Build history of the part. All positions in model axes, mm. A direction names the side the tool comes from. Give positions to 0.01 mm unless a question says otherwise; leave off trailing zeros. Write each loop counter-clockwise with the first axis right and the second up, starting at its lowest first coordinate (ties: lowest second). Pieces come first, ordered by that corner, then holes. Notation, with made-up numbers: (-12.5, 64) -> (4.5, 64) arc R22 ccw to (4.5, 73) -> close; hole circle Ø1 at (52, -27.5). An arc over 180 degrees is marked (long way). Write item = value, one per line. Start each with the question number.
Q1. Saw through at A-A, the plane y = 2. List the corners of the cut face in (x, z).
Q2. Drop flat-ended pins along their axis: P1, Ø5, axis at y = 3.5, z = -31, coming from the +X side; P2, Ø5, axis at y = 2.5, z = -21.5, coming from the -X side; P3, Ø1.5, axis at x = -8, z = -12.5, coming from the -Y side. Give the stop position or say it passes through.
Q3. Tool access for faces 1 (the face through (-5.26, 11.52, -18.68)), 2 (the face through (-20, 5, -3)), 3 (the face through (-42.05, 4.93, -3.43)), 4 (the face through (-36.238, 1.479, -29.956)), 5 (the face through (-42.07, 4.93, -46.55)): list every direction of +Z, -Z, +X, -X, +Y, -Y with a clear straight run to the whole face (end or side of a thin tool).
Q4. Mould opens along X. For faces 6 (the face through (-29.04, 1.48, -8.59)), 7 (the face through (-43.45, 11.52, -48)), 8 (the face through (-15, 13, -9)) say: pulls with the +X half, pulls with the -X half, needs draft (parallel to the pull), parting line crosses it, or undercut.
Q5. Wall check: line 1 (X direction, y = 3.25, z = -25); line 2 (Z direction, x = -20.5, y = 12.2); line 3 (Z direction, x = -20.5, y = 5.5). Give the ranges that are in metal, low to high.
Q6. Saw through at D-D, the plane y = 7. List the corners of the cut face in (x, z).
Q7. Saw through at B-B, the plane x = -20.5. List the corners of the cut face in (y, z), then the cut area to 3 significant figures.
Q8. Saw through at C-C, the plane z = -25. List the corners of the cut face in (x, y).
Autodesk Inventor part; units mm, degrees
ref_plane "YZ Plane" through (0, 0, 0) normal (1, 0, 0) x (0, 1, 0)
ref_plane "XZ Plane" through (0, 0, 0) normal (0, 1, 0) x (-1, 0, 0)
ref_plane "XY Plane" through (0, 0, 0) normal (0, 0, 1) x (1, 0, 0)
sketch "Эскиз1" plane through (0, 0, 0) normal (0, 1, 0) x (-1, 0, 0)
  arc A0 (41, -50) -> (45.5, -45.5) centre (41, -45.5) ccw
  line L0 (0, -50) -> (41, -50)
  arc A1 (-4.5, -45.5) -> (0, -50) centre (0, -45.5) ccw
  line L1 (-4.5, -4.5) -> (-4.5, -45.5)
  arc A2 (0, 0) -> (-4.5, -4.5) centre (0, -4.5) ccw
  line L2 (-1.5, -45.5) -> (-1.5, -4.5)
  arc A3 (0, -3) -> (-1.5, -4.5) centre (0, -4.5) ccw
  line L3 (0, -3) -> (41, -3)
  line L4 (41, 0) -> (0, 0)
  arc A4 (45.5, -4.5) -> (41, 0) centre (41, -4.5) ccw
  line L5 (45.5, -45.5) -> (45.5, -4.5)
  line L6 (42.5, -4.5) -> (42.5, -45.5)
  arc A5 (42.5, -4.5) -> (41, -3) centre (41, -4.5) ccw
  line L7 (41, -47) -> (0, -47)
  arc A6 (41, -47) -> (42.5, -45.5) centre (41, -45.5) ccw
  arc A7 (-1.5, -45.5) -> (0, -47) centre (0, -45.5) ccw
  circle A8 centre (20.5, -25) radius 18.5
  circle A9 centre (20.5, -25) radius 16.5
  circle A10 centre (20.5, -25) radius 14.5
  circle A11 centre (20.5, -25) radius 13.5
  point P0 (11.5, -30)
extrude "Выдавливание1" add sketch "Эскиз1" along normal blind 10 contours L2 A3 L3 A5 L6 A6 L7 A7 | A8 | A9 | A10 | A11
extrude "Выдавливание2" cut sketch "Эскиз1" along normal blind 3 contours A8 | A10
extrude "Выдавливание3" cut sketch "Эскиз1" along normal blind 14.75 contours A10 | A11
extrude "Выдавливание4" add sketch "Эскиз1" along normal blind 13 contours L0 A1 L1 A2 L4 A4 L5 A0
extrude "Выдавливание5" add sketch "Эскиз1" along normal blind 13 contours L2 A3 L3 A5 L6 A6 L7 A7 | A8 | A9 | A10 | A11
extrude "Выдавливание6" cut sketch "Эскиз1" along normal blind 10 contours L0 A1 L1 A2 L4 A4 L5 A0
extrude "Выдавливание7" cut sketch "Эскиз1" along normal blind 3 contours A8 | A10
extrude "Выдавливание8" cut sketch "Эскиз1" along normal blind 15 contours A10 | A11
sketch "Эскиз2" plane through (0, 13, 0) normal (0, 1, 0) x (1, 0, 0)
  circle A0 centre (-20.5, 25) radius 14.5
  line L0 (-45.5, 45.5) -> (-45.5, 4.5)
  arc A1 (-45.5, 4.5) -> (-41, 0) centre (-41, 4.5) ccw
  line L1 (-41, 0) -> (0, 0)
  arc A2 (0, 0) -> (4.5, 4.5) centre (0, 4.5) ccw
  line L2 (4.5, 4.5) -> (4.5, 45.5)
  arc A3 (4.5, 45.5) -> (0, 50) centre (0, 45.5) ccw
  line L3 (0, 50) -> (-41, 50)
  arc A4 (-41, 50) -> (-45.5, 45.5) centre (-41, 45.5) ccw
  circle A5 centre (-20.5, 25) radius 16.5
extrude "Выдавливание9" cut sketch "Эскиз2" against normal blind 3 contours A5
sketch "Эскиз3" plane through (0, 13, 0) normal (0, 1, 0) x (1, 0, 0)
  circle A0 centre (-20.5, 25) radius 16.5
  line L0 (-45.5, 45.5) -> (-45.5, 4.5)
  arc A1 (-45.5, 4.5) -> (-41, 0) centre (-41, 4.5) ccw
  line L1 (-41, 0) -> (0, 0)
  arc A2 (0, 0) -> (4.5, 4.5) centre (0, 4.5) ccw
  line L2 (4.5, 4.5) -> (4.5, 45.5)
  arc A3 (4.5, 45.5) -> (0, 50) centre (0, 45.5) ccw
  line L3 (0, 50) -> (-41, 50)
  arc A4 (-41, 50) -> (-45.5, 45.5) centre (-41, 45.5) ccw
  line L4 (-41, 49) -> (0, 49)
  arc A5 (3.5, 45.5) -> (0, 49) centre (0, 45.5) ccw
  line L5 (3.5, 45.5) -> (3.5, 4.5)
  arc A6 (0, 1) -> (3.5, 4.5) centre (0, 4.5) ccw
  line L6 (0, 1) -> (-41, 1)
  arc A7 (-44.5, 4.5) -> (-41, 1) centre (-41, 4.5) ccw
  line L7 (-44.5, 4.5) -> (-44.5, 45.5)
  arc A8 (-41, 49) -> (-44.5, 45.5) centre (-41, 45.5) ccw
  dimension "d18" = 1
extrude "Выдавливание10" cut sketch "Эскиз3" against normal blind 3 contours A4 L3 A3 L2 A2 L1 A1 L0
properties part number "Cap_top" material "Стекло, литое, серое"
Report:
q1.outline = (-42.5, -45.5) arc R1.5 ccw to (-41, -47) -> (0, -47) arc R1.5 ccw to (1.5, -45.5) -> (1.5, -4.5) arc R1.5 ccw to (0, -3) -> (-41, -3) arc R1.5 ccw to (-42.5, -4.5) -> close; circle Ø33 at (-20.5, -25); hole circle Ø37 at (-20.5, -25); hole circle Ø29 at (-20.5, -25)
q2.P1 = 1.5
q2.P2 = -42.5
q2.P3 = 3
q3.face_1 = +Y
q3.face_2 = +Z, +X, -X, -Y
q3.face_3 = +Z, -X, -Y
q3.face_4 = -Y
q3.face_5 = -Z, -X, -Y
q4.face_6 = undercut
q4.face_7 = pulls with the -X half
q4.face_8 = needs draft
q5.line_1 = -42.5 to -35, -6 to 1.5
q5.line_2 = -49 to -41.5, -8.5 to -1
q5.line_3 = -47 to -39.5, -10.5 to -3
q6.outline = (-42.5, -45.5) arc R1.5 ccw to (-41, -47) -> (0, -47) arc R1.5 ccw to (1.5, -45.5) -> (1.5, -4.5) arc R1.5 ccw to (0, -3) -> (-41, -3) arc R1.5 ccw to (-42.5, -4.5) -> close; hole circle Ø29 at (-20.5, -25)
q7.outline = (0, -47) -> (10, -47) -> (10, -49) -> (13, -49) -> (13, -41.5) -> (10, -41.5) -> (10, -39.5) -> (0, -39.5) -> (0, -41.5) -> (3, -41.5) -> (3, -43.5) -> (0, -43.5) -> close; (0, -10.5) -> (10, -10.5) -> (10, -8.5) -> (13, -8.5) -> (13, -1) -> (10, -1) -> (10, -3) -> (0, -3) -> (0, -6.5) -> (3, -6.5) -> (3, -8.5) -> (0, -8.5) -> close
q7.area = 183 mm2
q8.outline = (-44.5, 10) -> (-42.5, 10) -> (-42.5, 0) -> (-39, 0) -> (-39, 3) -> (-37, 3) -> (-37, 0) -> (-35, 0) -> (-35, 10) -> (-37, 10) -> (-37, 13) -> (-44.5, 13) -> close; (-6, 0) -> (-4, 0) -> (-4, 3) -> (-2, 3) -> (-2, 0) -> (1.5, 0) -> (1.5, 10) -> (3.5, 10) -> (3.5, 13) -> (-4, 13) -> (-4, 10) -> (-6, 10) -> close
